Verification items for this drawing (mm, ordinates from the low corner). Coordinates: 2 decimals unless noted, no trailing zeros. Order: outer loops, then holes, each group sorted by start corner. A loop starts at its lowest first (then second) coordinate and runs counter-clockwise, first axis right, second up. Notation, with made-up numbers: (81.5, -32) -> (126.5, -32) arc R11 ccw to (126.5, -24) -> close; hole circle Ø1 at (40, 66.25). An arc over 180 degrees is marked (long way). Write each question's results on one line, items separated by ' | '. Start each with the question number.
(1) Thickness scan on probe 1 along X at (y, z) = (74.5, 2.05); probe 2 along X at (y, z) = (44, 0.9). Record the ranges inside material, lowest first. Write a range as [from, to].
(2) Go/stop test with flat-tipped pins: pin 1 (3 mm diameter, centred on x = 34.5, y = 66.5, fed in from -Z); pin 2 (0.9 mm diameter, centred on y = 87, z = 2, fed in from -X); pin 3 (1.5 mm diameter, centred on x = 83, z = 1.5, fed in from -Y); pin 4 (0.9 mm diameter, centred on y = 23.5, z = 2, fed in from +X). Record where each tip stops, or that it passes through.
(3) Cross-section at C-C on y = 31.5. Enter the section's corners in (x, z).
(4) Cross-section at B-B on x = 17. Enter the section's corners in (y, z).
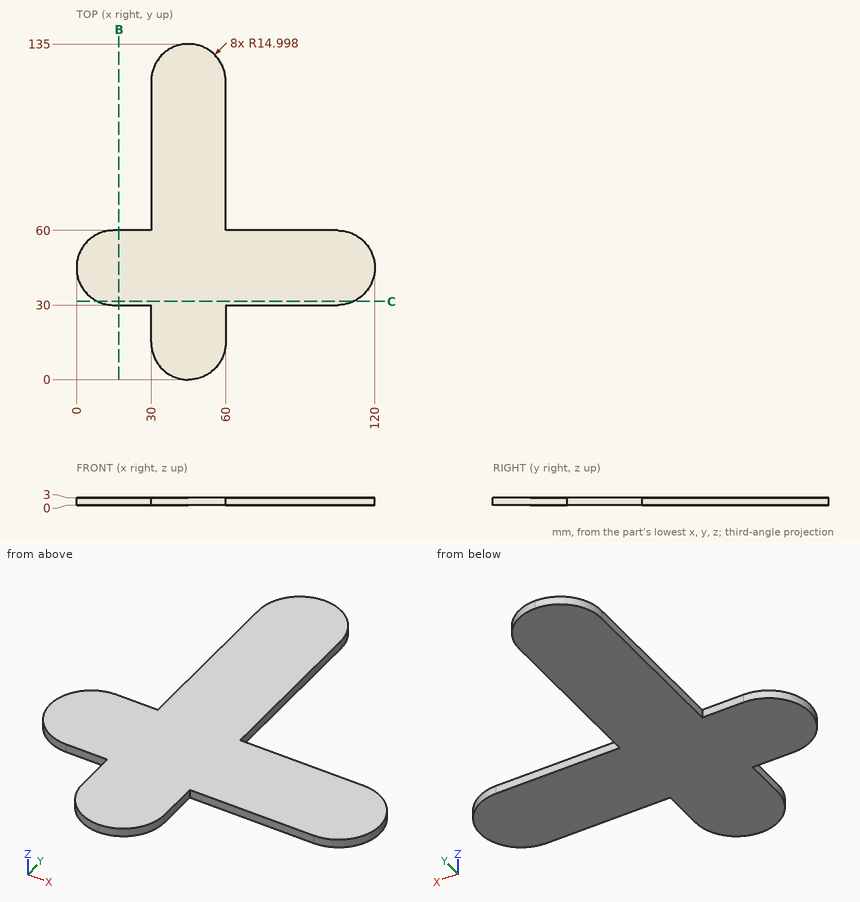
Results are:
1) probe 1: x = [30, 60] | probe 2: x = [0.03, 119.97]
2) pin 1: stops at z = 0 | pin 2: stops at x = 30 | pin 3: stops at y = 30 | pin 4: stops at x = 60
3) outline: (8.46, 0) -> (111.54, 0) -> (111.54, 3) -> (8.46, 3) -> close
4) outline: (30, 0) -> (60, 0) -> (60, 3) -> (30, 3) -> close
